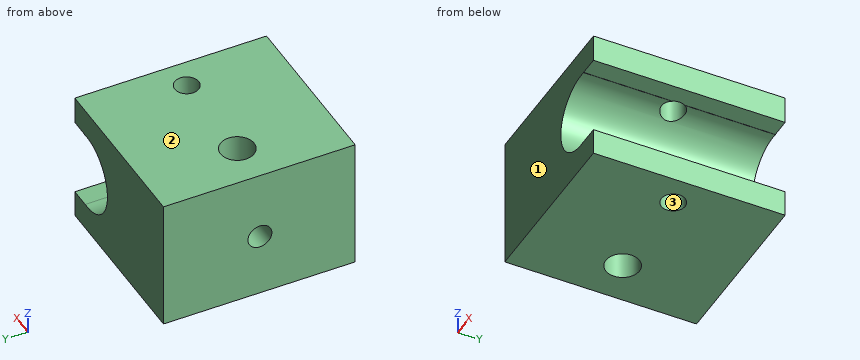
from build123d import *

# Parameters (mm, degrees)
F0_W     = 18
F0_H     = 14
F1_DEPTH = 20
F3_DEPTH = 20
F4_R     = 1.25
F4_R_2   = 1.75
F5_DEPTH = 25
F6_R     = 1.25
F7_DEPTH = 25


with BuildPart() as f1:
    # F0 (on Front) → F1 (new body)
    with BuildSketch(Plane.XZ):
        with Locations((4.047778, 20.754311)):
            Rectangle(F0_W, F0_H)
    extrude(amount=F1_DEPTH)

    # F2 (on face) → F3 (cut)
    with BuildSketch(Plane.XZ.offset(20)):
        with BuildLine():
            Line((13.047778, 17.367337), (13.047778, 24.034069))
            ThreePointArc((13.047778, 24.034069), (12.099173, 24.560953), (11.046412, 24.823921))
            ThreePointArc((11.046412, 24.823921), (6.426039, 20.753776), (10.940806, 16.566795))
            ThreePointArc((10.940806, 16.566795), (12.049681, 16.821286), (13.047778, 17.367337))
        make_face()
        with BuildLine():
            Line((13.047778, 16.563023), (13.047778, 17.367337))
            ThreePointArc((13.047778, 17.367337), (12.049681, 16.821286), (10.940806, 16.566795))
            Line((10.940806, 16.566795), (13.047778, 16.563023))
        make_face()
        with BuildLine():
            ThreePointArc((11.046412, 24.823921), (12.099173, 24.560953), (13.047778, 24.034069))
            Line((13.047778, 24.034069), (13.047778, 24.851898))
            Line((13.047778, 24.851898), (11.046412, 24.851898))
            Line((11.046412, 24.851898), (11.046412, 24.823921))
        make_face()
    extrude(amount=-F3_DEPTH, mode=Mode.SUBTRACT)

    # F4 (on face) → F5 (cut)
    with BuildSketch(Plane.XY.offset(27.754311)):
        with Locations((9.971282, -10.096995)):
            Circle(F4_R)
        with Locations((-0.444201, -10.021016)):
            Circle(F4_R_2)
    extrude(amount=-F5_DEPTH, mode=Mode.SUBTRACT)

    # F6 (on face) → F7 (cut)
    with BuildSketch(Plane(origin=(-4.952222, 0, 0), x_dir=(0, -1, 0), z_dir=(-1, 0, 0))):
        with Locations((10.059365, 20.492349)):
            Circle(F6_R)
    extrude(amount=-F7_DEPTH, mode=Mode.SUBTRACT)


solid = f1.part
Part model, mm, in its own coordinate system. Face numbers are marked on the shaded views. Round coordinates to 2 decimals unless told otherwise and drop trailing zeros. Write each loop counter-clockwise with the first axis right and the second up, starting at its lowest first coordinate (ties: lowest second). Pieces come first, ordered by that corner, then holes. Notation, with made-up numbers: M -1,43.5 L 24,43.5 A16 ccw 24,50.5 Z; hole C 1.25,16.25 d3. An arc over 180 degrees is marked long. Return JSON: item names as keys, results as strings. Group by question number.
(1) Two-plate mould, pull along Y, no slides. Class the marked faces 1, 2 and 3: +Y half, -Y half, draft (parallel to the pull), parting line (faces both ways), or undercut.
(2) Saw through at B-B on x = 4. Write the cut outline in (y, z), then the cut area to 3 significant figures.
(3) Pin check, flat tip, straight feed: pin 1 Ø3 at (y, z) = (-10.06, 20.49) entering from +X. Stop position of the tip, or through.
(4) Drill centre lines: probe 1 along Z at (x, y) = (11.5, -4.75); probe 2 along Y at (x, z) = (10, 16); probe 3 along X at (y, z) = (-10.5, 23). Where is each one in solid material? Low to high.
(5) Saw through at C-C on z = 15.25. Write the cut outline in (x, y), then the cut area to 3 significant figures.
(6) Saw through at D-D on z = 17.25. Write the cut outline in (x, y).
Returned:
{
 "1": {"face 1": "-Y half", "face 2": "draft", "face 3": "undercut"},
 "2": {"outline": "M -20,13.75 L 0,13.75 L 0,27.75 L -20,27.75 Z; hole C -10.06,20.49 d2.5", "area": "275 mm²"},
 "3": {"pin 1": "x = 6.79"},
 "4": {"probe 1": "13.75 to 16.57, 24.85 to 27.75", "probe 2": "-20 to -11.35, -8.85 to 0", "probe 3": "-4.95 to -2.13, 1.24 to 7.12"},
 "5": {"outline": "M -4.95,-20 L 13.05,-20 L 13.05,0 L -4.95,0 Z; hole C -0.44,-10.02 d3.5; hole C 9.97,-10.1 d2.5", "area": "345 mm²"},
 "6": {"outline": "M -4.95,-20 L 8.27,-20 L 8.27,0 L -4.95,0 Z; hole C -0.44,-10.02 d3.5"}
}
